```python
from build123d import *

# Parameters (mm, degrees)
F1_DEPTH    = 20
F3_D        = 6.6
F5_D        = 11
F5_DEPTH    = 6.4
F5_TIP      = 3.3047334047
F7_D        = 11
F7_DEPTH    = 6.4
F7_TIP      = 3.3047334047
F8_T1_DEPTH = 21.6433659759
F8_T3_DEPTH = 25.1433659759
F8_T5_DEPTH = 21.6433659759
F8_T7_DEPTH = 25.0580427678
F9_SIZE     = 0.5


# Not quite as in the source:
# - a fillet or chamfer that OpenCascade refuses, or shapes differently, is made with other operations: its cross-section is extruded or revolved along the edge and cut away or added


with BuildPart() as f1:
    # F0 (on Front) → F1 (new body)
    with BuildSketch(Plane.XZ):
        with BuildLine():
            ThreePointArc((-27.5, 0), (0, 27.5), (27.5, 0))
            Line((27.5, 0), (44, 0))
            Line((44, 0), (44, 24))
            Line((44, 24), (30, 24))
            Line((30, 24), (17.5, 38))
            Line((17.5, 38), (-17.5, 38))
            Line((-17.5, 38), (-30, 24))
            Line((-30, 24), (-44, 24))
            Line((-44, 24), (-44, 0))
            Line((-44, 0), (-27.5, 0))
        make_face()
    extrude(amount=F1_DEPTH)

    # F3 (through all)
    with Locations(Plane(origin=(0, 0, 0), x_dir=(1, 0, 0), z_dir=(0, 0, -1))):
        with Locations((-35.5, 10), (35.5, 10)):
            Hole(F3_D / 2)

    # F5
    with Locations(Plane.XY.offset(24)):
        with Locations((-35.5, -10)):
            Hole(F5_D / 2, depth=F5_DEPTH)
            with Locations((0, 0, -(F5_DEPTH + F5_TIP / 2))):  # 118° drill point
                Cone(0, F5_D / 2, F5_TIP, mode=Mode.SUBTRACT)

    # F7
    with Locations(Plane.XY.offset(24)):
        with Locations((35.5, -10)):
            Hole(F7_D / 2, depth=F7_DEPTH)
            with Locations((0, 0, -(F7_DEPTH + F7_TIP / 2))):  # 118° drill point
                Cone(0, F7_D / 2, F7_TIP, mode=Mode.SUBTRACT)

    # F8: chamfer of 1 on 8 edges, made by hand

    # F8_s2 → F8_t1 (cut)
    with BuildSketch(Plane.YZ.offset(24.928317012)):
        Polygon((-19, 0), (-20, 1), (-20, 0), align=None)
        Polygon((-1, 0), (0, 1), (0, 0), align=None)
    extrude(amount=F8_T1_DEPTH, mode=Mode.SUBTRACT)

    # F8_s4 → F8_t3 (cut)
    with BuildSketch(Plane.XZ.offset(-2.571682988)):
        Polygon((43, 0), (44, 1), (44, 0), align=None)
        Polygon((-43, 0), (-44, 1), (-44, 0), align=None)
    extrude(amount=F8_T3_DEPTH, mode=Mode.SUBTRACT)

    # F8_s6 → F8_t5 (cut)
    with BuildSketch(Plane.YZ.offset(-46.571682988)):
        Polygon((-19, 0), (-20, 1), (-20, 0), align=None)
        Polygon((-1, 0), (0, 1), (0, 0), align=None)
    extrude(amount=F8_T5_DEPTH, mode=Mode.SUBTRACT)

    # F8_s8 → F8_t7 (cut)
    with BuildSketch(Plane.XZ.offset(-2.5290213839)):
        with BuildLine():
            Line((-27.4830665009, 0.9649122807), (-28.4824507373, 0))
            Line((-28.4824507373, 0), (-27.5, 0))
            ThreePointArc((-27.5, 0), (-27.4955143469, 0.4966797747), (-27.4830665009, 0.9649122807))
        make_face()
        with BuildLine():
            Line((27.4830665009, 0.9649122807), (28.4824507373, 0))
            Line((28.4824507373, 0), (27.5, 0))
            ThreePointArc((27.5, 0), (27.4955143469, 0.4966797747), (27.4830665009, 0.9649122807))
        make_face()
    extrude(amount=F8_T7_DEPTH, mode=Mode.SUBTRACT)

    # F9
    f9_edges = [f1.edges().sort_by_distance(p)[0] for p in [
        (44, -20, 12.5),
        (44, 0, 12.5),
        (44, -10, 24),
        (37, -20, 24),
        (37, 0, 24),
        (23.75, 0, 31),
        (23.75, -20, 31),
        (0, -20, 38),
        (0, 0, 38),
        (-23.75, -20, 31),
        (0, -20, 27.5),
        (-44, -20, 12.5),
        (-37, -20, 24),
        (-44, -10, 24),
        (-37, 0, 24),
        (0, 0, 27.5),
        (-23.75, 0, 31),
        (-44, 0, 12.5),
    ]]
    chamfer(f9_edges, length=F9_SIZE)


solid = f1.part
```
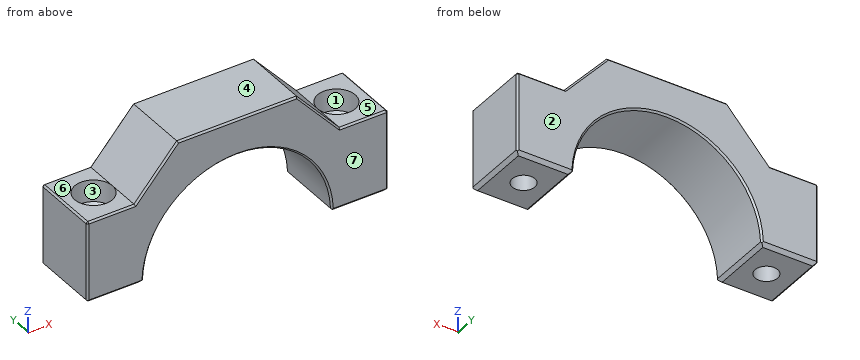
Model file for the job. Use its own axes, mm. Face numbers are marked on the shaded views. A direction names the side the tool comes from. Coordinates: 2 decimals unless noted, no trailing zeros. Loops run counter-clockwise (first coordinate to the right, second up) from the corner with the lowest first, then second, coordinate; pieces in that order, holes last. Notation, with made-up numbers: (-23.75, -38) - (18.25, -38) arc R21 cw to (18.25, -20) - close; hole circle Ø4 at (74, 47). An arc over 180 degrees is marked (long way). Answer as a JSON object with one key per item and string values. Group by question number.
(1) Cut at D-D (z = 30). Give the cut face in (x, y), then the cut area to 3 significant figures.
(2) Cut at B-B (x = 0). Give the cut face in (y, z).
(3) Cut at C-C (z = 10). State how many separate pieces and enclosed holes the cut face has, then the cut area to 3 significant figures.
(4) Tool access for the marked faces 5, 6 and 7: list every direction of +Z, -Z, +X, -X, +Y, -Y with a clear straight run to the whole face (end or side of a thin tool).
(5) Flat gauge pins, fed straight in: pin 1 (6.5 mm diameter, centred on x = 35.5, y = -10, fed in from +Z); pin 2 (2 mm diameter, centred on x = 31.5, y = -7, fed in from +Z); pin 3 (1.5 mm diameter, centred on x = 12.5, y = -4, fed in from -Z). Where does each tip first touch, or does it go through?
(6) Probe line 1 along Y through (x, z) = (-35.5, 20.75); line 2 along X through (y, z) = (-10, 11.5); line 3 along X through (y, z) = (-10, 7.5). List the from-to ranges inside material, lowest first.
(7) Cut at A-A (x = -35.5). Give the cut face in (y, z), then the cut area to 3 significant figures.
(8) Two-plate mould, pull along Y, no slides. Class the marked faces 1, 2, 3 and 4: released by +Y, released by -Y, zero draft, split by the parting line, or undercut.
Geometry says:
{
 "1": {"outline": "(-24.64, -19.5) - (-23.97, -20) - (23.97, -20) - (24.64, -19.5) - (24.64, -0.5) - (23.97, 0) - (-23.97, 0) - (-24.64, -0.5) - close", "area": "985 mm^2"},
 "2": {"outline": "(-20, 28) - (-19.5, 27.5) - (-0.5, 27.5) - (0, 28) - (0, 37.5) - (-0.5, 38) - (-19.5, 38) - (-20, 37.5) - close"},
 "3": {"separate pieces": "2", "enclosed holes": "2", "area": "666 mm^2"},
 "4": {"face 5": "+Z, +X, +Y, -Y", "face 6": "+Z, -X, +Y, -Y", "face 7": "+Z, -Z, +X, -X, -Y"},
 "5": {"pin 1": "passes through", "pin 2": "stops at z = 24", "pin 3": "stops at z = 24.1"},
 "6": {"line 1": "y = -20 to -15.5, -4.5 to 0", "line 2": "x = -44 to -38.8, -32.2 to -24.98, 24.98 to 32.2, 38.8 to 44", "line 3": "x = -44 to -38.8, -32.2 to -26.46, 26.46 to 32.2, 38.8 to 44"},
 "7": {"outline": "(-20, 1) - (-19, 0) - (-13.3, 0) - (-13.3, 16.28) - (-15.5, 17.6) - (-15.5, 24) - (-19.5, 24) - (-20, 23.5) - close; (-6.7, 0) - (-1, 0) - (0, 1) - (0, 23.5) - (-0.5, 24) - (-4.5, 24) - (-4.5, 17.6) - (-6.7, 16.28) - close", "area": "289 mm^2"},
 "8": {"face 1": "undercut", "face 2": "released by +Y", "face 3": "undercut", "face 4": "zero draft"}
}
